Autodesk Inventor part; units mm, degrees
ref_plane "YZ Plane" through (0, 0, 0) normal (1, 0, 0) x (0, 1, 0)
ref_plane "XZ Plane" through (0, 0, 0) normal (0, 1, 0) x (-1, 0, 0)
ref_plane "XY Plane" through (0, 0, 0) normal (0, 0, 1) x (1, 0, 0)
sketch "Sketch1" plane through (0, 0, 0) normal (0, 0, 1) x (1, 0, 0)
  circle A0 centre (0, 0) radius 17.5
  line L0 (-15.1554, -8.75) -> (-13.6554, -11.3481)
  line L1 (-15.1554, -8.75) -> (-16.6554, -6.1519)
  line L2 (-16.6554, -6.1519) -> (-19.2535, -7.6519)
  line L3 (-19.2535, -7.6519) -> (-16.2535, -12.8481)
  line L4 (0, 0) -> (0, -17.5)
  line L5 (0, 0) -> (15.1554, -8.75)
  line L6 (0, 0) -> (17.5, 0) construction
  line L7 (0, 0) -> (17.5, 0) construction
  line L8 (0, 17.5) -> (0, -17.5)
  line L9 (-15.1554, -8.75) -> (0, 0)
  line L10 (0, -17.5) -> (3, -17.5)
  line L11 (3, -17.5) -> (3, -20.5)
  line L12 (-3, -17.5) -> (0, -17.5)
  arc A1 (-16.2535, -12.8481) -> (-3, -20.5) centre (0, 0) ccw
  line L13 (-3, -17.5) -> (-3, -14)
  line L14 (-3, -10.5) -> (3, -10.5)
  line L15 (3, -10.5) -> (3, -17.5)
  arc A2 (-3, -10.5) -> (-9.5308, -14.9804) centre (-3, -17.5) ccw
  arc A3 (-3, -14) -> (-5.4652, -19.9845) centre (-3, -17.5) ccw
  arc A4 (-13.6554, -11.3481) -> (-9.5308, -14.9804) centre (0, 0) ccw
  arc A5 (-6.3746, -16.5715) -> (-3, -17.5) centre (0, 0) ccw
  point P0 (0, -10.5)
  point P1 (-3, -17.2409)
  point P2 (3, -17.2409)
  dimension "d0" = 35
  dimension "d1" = 3
  dimension "d2" = 3
  dimension "d3" = 3
  dimension "d4" = 330
  dimension "d6" = 35
  dimension "d8" = 3
  dimension "d9" = 3
  dimension "d10" = 6
  dimension "d11" = 3
  dimension "d29" = 7
  dimension "d30" = 6
extrude "Extrusion1" add sketch "Sketch1" along normal blind 12 contours L0 A4 A2 A0 A3 A1 L3 L2 L1 | L15 L10 A0 | A0 L4 L14 L15 | A2 L14 L4 A0 L13 A3 | L12 L13 A0
sketch "Sketch2" plane through (-16.6554, -6.1519, 12) normal (0.866, 0.5, 0) x (0, 0, -1)
  line L0 (0, 0) -> (0, -3)
  line L1 (12, -6) -> (0, -6)
  line L2 (0, -3) -> (12, -3)
  line L3 (0, -3) -> (3, -3)
  line L4 (3, -3) -> (9, -3)
  circle A0 centre (3, -3) radius 1.5
  circle A1 centre (9, -3) radius 1.5
  dimension "d14" = 3
  dimension "d15" = 3
  dimension "d16" = 6
  dimension "d17" = 3
  dimension "d18" = 3
extrude "Extrusion2" cut sketch "Sketch2" against normal blind 12
sketch "Sketch3" plane through (-3, -17.5, 0) normal (0, -1, 0) x (1, 0, 0)
  line L0 (6, 12) -> (0, 12)
  line L1 (3, 0) -> (3, 3)
  line L2 (3, 3) -> (3, 9)
  circle A0 centre (3, 3) radius 1.5
  circle A1 centre (3, 9) radius 1.5
  dimension "d23" = 3
  dimension "d24" = 6
  dimension "d25" = 3
  dimension "d26" = 3
extrude "Extrusion3" cut sketch "Sketch3" against normal blind 12
fillet "Fillet1" radius 2 1 edges at (-5.4652, -19.9845, 6)
properties part number "acople" material "Iron, Ductile"
Verification items for the finished model (mm, model axes). A direction names the side the tool comes from. Coordinates: 2 decimals unless noted, no trailing zeros. Loops run counter-clockwise (first coordinate to the right, second up) from the corner with the lowest first, then second, coordinate; pieces in that order, holes last. Notation, with made-up numbers: (56, -15) - (114, -15) arc R19 ccw to (114, 16) - close; hole circle Ø11 at (74.5, 82). An arc over 180 degrees is marked (long way). Return JSON: item names as keys, results as strings.
1. Section check C-C, the plane x = -4. Record the boundary of the cut face in (y, z).
Established:
{"outline": "(-14.15, 0) - (-10.57, 0) - (-10.57, 12) - (-14.15, 12) - close"}
2. Section check B-B, the plane z = 7.75. Count the separate pieces of the cut face and the enclosed holes in it, then the cut area to 3 significant figures.
Established:
{"separate pieces": "3", "enclosed holes": "0", "area": "95.5 mm2"}
3. Mould release check, pull along Y, two halves, no side actions. Record for faces 1 (the flat face through (3, -14, 6)), 2 (the cylindrical face through (-16.149, -9.987, 7.614)), 3 (the flat face through (-17.775, -10.214, 5.916)): +Y half, -Y half, draft (parallel to the pull), parting line (faces both ways), or undercut.
Established:
{"face 1": "draft", "face 2": "undercut", "face 3": "-Y half"}
4. Go/stop test with flat-tipped pins: pin 1 (6.5 mm diameter, centred on x = 1, z = 7.5, fed in from -Y); pin 2 (1 mm diameter, centred on y = -15.5, z = 4, fed in from -X); pin 3 (3 mm diameter, centred on y = -15, z = 8.5, fed in from -X). Record where each tip stops, or that it passes through.
Established:
{"pin 1": "stops at y = -17.5", "pin 2": "stops at x = -14.29", "pin 3": "stops at x = -15.72"}
5. Section check A-A, the plane x = 0. Record the boundary of the cut face in (y, z).
Established:
{"outline": "(-17.5, 0) - (-10.5, 0) - (-10.5, 1.5) - (-17.5, 1.5) - close; (-17.5, 4.5) - (-10.5, 4.5) - (-10.5, 7.5) - (-17.5, 7.5) - close; (-17.5, 10.5) - (-10.5, 10.5) - (-10.5, 12) - (-17.5, 12) - close"}
6. Thickness scan on L1, parallel to Z at x = 0, y = -15.75; L2, parallel to X at y = -14.75, z = 3; L3, parallel to X at y = -11.75, z = 3.5. Record the ranges inside material, lowest first.
Established:
{"L1": "z = 0 to 1.5, 4.5 to 7.5, 10.5 to 12", "L2": "x = -14.55 to -9.88, -9.44 to -5.17, -3 to -1.5, 1.5 to 3", "L3": "x = -16.89 to -13.31, -6.99 to -1.41, 1.41 to 3"}
7. Tool access check on faces 4 (the cylindrical face through (-11.705, -13.35, 5.916)), 5 (the flat face through (-3, -16, 6)), 6 (the flat face through (0, -17.5, 6)), 7 (the flat face through (0, -10.5, 6)). Record the directions out of +Z, -Z, +X, -X, +Y, -Y that give a thin tool (end or side, any length) a straight path to the whole face; none if there is none.
Established:
{"face 4": "+Z, -Z, +Y", "face 5": "+Z, -Z, -Y", "face 6": "+Z, -Z, +X, -Y", "face 7": "+Z, -Z, +X, +Y"}
